```python
from build123d import *

# Parameters (mm, degrees)
EXTRUDE_1_DEPTH     = 10
SKETCH_2_R          = 19
CUT_EXTRUDE_1_DEPTH = 8
CUT_EXTRUDE_2_DEPTH = 9
SKETCH_4_R          = 1.75
CUT_EXTRUDE_3_DEPTH = 31
SKETCH_5_R          = 3.1
CUT_EXTRUDE_4_DEPTH = 3.5
SKETCH_6_R          = 4
EXTRUDE_2_DEPTH     = 6


with BuildPart() as part:
    # Эскиз1 → Бобышка-Вытянуть1 (new body)
    with BuildSketch(Plane(origin=(0, 0, 0), x_dir=(1, 0, 0), z_dir=(0, 1, 0))):
        with BuildLine():
            Line((16, -20), (-16, -20))
            ThreePointArc((-16, -20), (-18.828427125, -18.828427125), (-20, -16))
            Line((-20, -16), (-20, 16))
            ThreePointArc((-20, 16), (-18.828427125, 18.828427125), (-16, 20))
            Line((-16, 20), (16, 20))
            ThreePointArc((16, 20), (18.828427125, 18.828427125), (20, 16))
            Line((20, 16), (20, -16))
            ThreePointArc((20, -16), (18.828427125, -18.828427125), (16, -20))
        make_face()
    extrude(amount=EXTRUDE_1_DEPTH)

    # Эскиз2 → Вырез-Вытянуть1 (cut)
    with BuildSketch(Plane(origin=(0, 10, 0), x_dir=(1, 0, 0), z_dir=(0, 1, 0))):
        with Locations(Location((0, 0, 0), (0, 0, 270))):
            Circle(SKETCH_2_R)
    extrude(amount=-CUT_EXTRUDE_1_DEPTH, mode=Mode.SUBTRACT)

    # Эскиз3 → Вырез-Вытянуть2 (cut)
    with BuildSketch(Plane(origin=(0, 2, 0), x_dir=(1, 0, 0), z_dir=(0, 1, 0))):
        with BuildLine():
            Line((-10, -4.582575695), (-10, -16.155494421))
            ThreePointArc((-10, -16.155494421), (-18.973695145, 0.999446125), (-8.247376329, 17.116681445))
            Line((-8.247376329, 17.116681445), (0.173394535, 10.998633294))
            ThreePointArc((0.173394535, 10.998633294), (-9.210540816, 6.013812257), (-10, -4.582575695))
        make_face()
        with BuildLine():
            Line((-6, -9.219544457), (-6, -18.027756377))
            ThreePointArc((-6, -18.027756377), (10.378017833, -15.915299113), (18.916407865, -1.780312749))
            Line((18.916407865, -1.780312749), (5.5, -9.526279442))
            ThreePointArc((5.5, -9.526279442), (-0.29329437, -10.996089233), (-6, -9.219544457))
        make_face()
        with BuildLine():
            Line((6.465637775, 8.899186938), (-6.067599609, 18.005116911))
            ThreePointArc((-6.067599609, 18.005116911), (10.850398881, 15.597078064), (18.991376746, 0.572371631))
            Line((18.991376746, 0.572371631), (9.977225575, -4.631950974))
            ThreePointArc((9.977225575, -4.631950974), (10.647293651, 2.763175331), (6.465637775, 8.899186938))
        make_face()
    extrude(amount=-CUT_EXTRUDE_2_DEPTH, mode=Mode.SUBTRACT)

    # Эскиз4 → Вырез-Вытянуть3 (cut, through all)
    with BuildSketch(Plane(origin=(0, 10, 0), x_dir=(1, 0, 0), z_dir=(0, 1, 0))):
        with Locations(Location((-16, 16, 0), (0, 0, 270))):
            Circle(SKETCH_4_R)
        with Locations(Location((16, 16, 0), (0, 0, 270))):
            Circle(SKETCH_4_R)
        with Locations(Location((-16, -16, 0), (0, 0, 270))):
            Circle(SKETCH_4_R)
        with Locations(Location((16, -16, 0), (0, 0, 270))):
            Circle(SKETCH_4_R)
    extrude(amount=-CUT_EXTRUDE_3_DEPTH, mode=Mode.SUBTRACT)

    # Эскиз5 → Вырез-Вытянуть4 (cut)
    with BuildSketch(Plane(origin=(0, 10, 0), x_dir=(1, 0, 0), z_dir=(0, 1, 0))):
        with Locations(Location((-16, 16, 0), (0, 0, 270))):
            Circle(SKETCH_5_R)
        with Locations(Location((16, 16, 0), (0, 0, 270))):
            Circle(SKETCH_5_R)
        with Locations(Location((16, -16, 0), (0, 0, 270))):
            Circle(SKETCH_5_R)
        with Locations(Location((-16, -16, 0), (0, 0, 270))):
            Circle(SKETCH_5_R)
    extrude(amount=-CUT_EXTRUDE_4_DEPTH, mode=Mode.SUBTRACT)

    # Эскиз6 → Бобышка-Вытянуть2 (add)
    with BuildSketch(Plane(origin=(0, 2, 0), x_dir=(1, 0, 0), z_dir=(0, 1, 0))):
        with Locations(Location((0, 0, 0), (0, 0, 270))):
            Circle(SKETCH_6_R)
    extrude(amount=EXTRUDE_2_DEPTH)


solid = part.part
```
The model under review builds one solid part; all positions refer to its coordinate system, in mm. A direction names the side the tool comes from. Round coordinates to 2 decimals unless told otherwise and drop trailing zeros. Write each loop counter-clockwise with the first axis right and the second up, starting at its lowest first coordinate (ties: lowest second). Pieces come first, ordered by that corner, then holes.
(1) Mouldability with a two-part tool opening along Z and no side actions: class faces 4 (the flat face through (0, 0, 0)), 5 (the cylindrical face through (17.735, 3.296, -16.228)), 6 (the cylindrical face through (18.797, 4.93, -18.859)) as +Z half, -Z half, draft (parallel to the pull), parting line (faces both ways), or undercut.
(2) Wall thickness on L1, parallel to X at y = 6, z = 15; L2, parallel to X at y = 8.4, z = -16; L3, parallel to Z at x = -1.5, y = 3: over which ranges is each line inside the solid? List them lowest first.
(3) We need section D-D on y = 1. Give the boundary of the cut face in (x, z), and give its area (3 significant figures).
(4) Insertion check: pin 1 (5.5 mm diameter, centred on x = -16, z = 16, fed in from +Y); pin 2 (6 mm diameter, centred on x = 7.5, z = 6, fed in from +Y); pin 3 (6.5 mm diameter, centred on x = 0, z = -1.5, fed in from +Y). Each pin has a flat end and moves straight along its axis. Give the tip position at first contact, or say it passes through.
(5) We need section A-A on y = 7. Give the boundary of the cut face in (x, z).
(6) Machinability: for faces 1 (the flat face through (14.55, 1.01, 1.99)), 2 (the cylindrical face through (-19.026, 8.274, 15.328)), 3 (the flat face through (0, 5, 20)), which of the approach directions +Z, -Z, +X, -X, +Y, -Y give a long, thin tool a straight path to every point of the face, cutting with its end or side? Answer none if there is none.
(7) We need section C-C on z = 7.5. Give the boundary of the cut face in (x, y).
(8) We need section B-B on x = -0.5. Give the boundary of the cut face in (y, z).
Findings below:
1. face 4: draft
1. face 5: undercut
1. face 6: -Z half
2. L1: x = -20 to -17.44, -14.56 to -11.66, 11.66 to 14.56, 17.44 to 20
2. L2: x = -20 to -19.1, -12.9 to -10.25, 10.25 to 12.9, 19.1 to 20
2. L3: z = -20 to -18.94, -3.71 to 3.71, 18.94 to 20
3. outline: (-20, -16) arc R4 ccw to (-16, -20) - (16, -20) arc R4 ccw to (20, -16) - (20, 16) arc R4 ccw to (16, 20) - (-16, 20) arc R4 ccw to (-20, 16) - close; hole circle Ø3.5 at (-16, -16); hole circle Ø3.5 at (-16, 16); hole (-10, 4.58) - (-10, 16.16) arc R19 ccw to (-8.25, -17.12) - (0.17, -11) arc R11 cw to start; hole (-6.07, -18.01) arc R19 ccw to (18.99, -0.57) - (9.98, 4.63) arc R11 cw to (6.47, -8.9) - close; hole (-6, 9.22) arc R11 cw to (5.5, 9.53) - (18.92, 1.78) arc R19 ccw to (-6, 18.03) - close; hole circle Ø3.5 at (16, -16); hole circle Ø3.5 at (16, 16)
3. area: 881 mm2
4. pin 1: stops at y = 6.5
4. pin 2: stops at y = 2
4. pin 3: stops at y = 8
5. outline: (-20, -16) arc R4 ccw to (-16, -20) - (16, -20) arc R4 ccw to (20, -16) - (20, 16) arc R4 ccw to (16, 20) - (-16, 20) arc R4 ccw to (-20, 16) - close; circle Ø8 at (0, 0); hole circle Ø6.2 at (-16, -16); hole circle Ø6.2 at (-16, 16); hole circle Ø38 at (0, 0); hole circle Ø6.2 at (16, -16); hole circle Ø6.2 at (16, 16)
6. face 1: +Y, -Y
6. face 2: +Y
6. face 3: +Z, +X, -X, +Y, -Y
7. outline: (-20, 0) - (-17.46, 0) - (-17.46, 10) - (-20, 10) - close; (-10, 0) - (9.01, 0) - (9.01, 2) - (-10, 2) - close; (17.46, 0) - (20, 0) - (20, 10) - (17.46, 10) - close
8. outline: (0, -20) - (10, -20) - (10, -18.99) - (0, -18.99) - close; (0, -13.96) - (2, -13.96) - (2, -11.49) - (0, -11.49) - close; (0, -10.99) - (2, -10.99) - (2, -3.97) - (8, -3.97) - (8, 3.97) - (2, 3.97) - (2, 10.99) - (0, 10.99) - close; (0, 18.99) - (10, 18.99) - (10, 20) - (0, 20) - close
